Autodesk Inventor part; units mm, degrees
ref_plane "YZ Plane" through (0, 0, 0) normal (1, 0, 0) x (0, 1, 0)
ref_plane "XZ Plane" through (0, 0, 0) normal (0, 1, 0) x (-1, 0, 0)
ref_plane "XY Plane" through (0, 0, 0) normal (0, 0, 1) x (1, 0, 0)
sketch "Sketch1" plane through (0, 0, 0) normal (0, 1, 0) x (-1, 0, 0)
  line L0 (0, 225) -> (0, -225) construction
  line L1 (5, 225) -> (5, -225)
  line L2 (-5, -225) -> (-5, 225)
  arc A0 (5, 225) -> (-5, 225) centre (0, 225) ccw
  arc A1 (-5, -225) -> (5, -225) centre (0, -225) ccw
  circle A2 centre (0, 0) radius 2.5
  dimension "d0" = 450
  dimension "d1" = 10
  dimension "d2" = 5
extrude "Extrusion1" add sketch "Sketch1" along normal blind 10 contours L1 A1 L2 A0 | A2
sketch "Sketch2" plane through (0, 0, 0) normal (0, -1, 0) x (1, 0, 0)
  circle A0 centre (0, 0) radius 2.5
  dimension "d5" = 5
extrude "Extrusion2" add sketch "Sketch2" along normal blind 5
sketch "Sketch3" plane through (0, 10, 0) normal (0, 1, 0) x (1, 0, 0)
  line L0 (-5, 225) -> (-5, -225)
  arc A0 (-5, -225) -> (5, -225) centre (0, -225) ccw
  line L1 (5, -225) -> (5, 225)
  arc A1 (5, 225) -> (-5, 225) centre (0, 225) ccw
  circle A2 centre (0, -225) radius 5
  circle A3 centre (0, 225) radius 5
  line L2 (-5, -230) -> (5, -230)
  line L3 (5, -230) -> (5, -220)
  line L4 (5, -220) -> (-5, -220)
  line L5 (-5, -220) -> (-5, -230)
  line L6 (-5, 225) -> (-5, -225)
  line L7 (-5, 220) -> (5, 220)
  line L8 (5, 220) -> (5, 230)
  line L9 (5, 230) -> (-5, 230)
  line L10 (-5, 230) -> (-5, 220)
  point P0 (0, 0)
  point P1 (5, 225)
  point P2 (5, -225)
  point P3 (-5, -225)
  point P4 (0, 230)
  point P5 (5, 225)
  point P6 (-5, -225)
  point P7 (0, -230)
  point P8 (5, -225)
  dimension "d8" = 10
  dimension "d9" = 10
extrude "Extrusion3" add sketch "Sketch3" against normal blind 20 contours L10 L9 A1 | A1 A3 | L9 L8 A1 | A2 A0 | A0 L2 L5 | A0 L3 L2
properties part number "McCrea_otočka_walle"
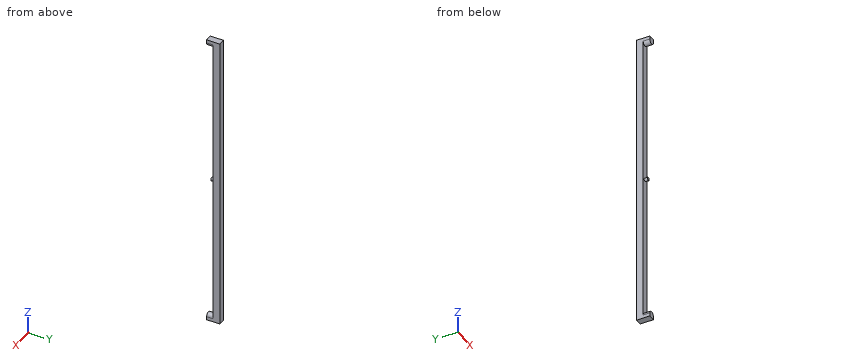
CAD build for the part. Positions are in the model's coordinates, mm. Round coordinates to 2 decimals unless told otherwise and drop trailing zeros. Order: outer loops, then holes, each group sorted by start corner. A loop starts at its lowest first (then second) coordinate and runs counter-clockwise, first axis right, second up.
Item 1: Probe line 1 along Y through (x, z) = (3, -87.5); line 2 along Z through (x, y) = (-2.25, -0.75); line 3 along Z through (x, y) = (4, -8.5). List the from-to ranges inside material, lowest first.
Item 2: Saw through at A-A on x = 0. Write the cut outline in (y, z).
Item 3: Saw through at B-B on z = 52. Write the cut outline in (x, y).
Item 4: Pin check, flat tips, straight feed: pin 1 (5 mm diameter, centred on x = -0.5, z = 27, fed in from -Y); pin 2 (2.5 mm diameter, centred on x = -1, z = 1, fed in from -Y). Stop position of each tip, or through.
Reported:
1. line 1: y = 0 to 10
1. line 2: z = -230 to -220.53, -1.09 to 1.09, 220.53 to 230
1. line 3: z = -230 to -222, 222 to 230
2. outline: (-10, -230) - (10, -230) - (10, 230) - (-10, 230) - (-10, 220) - (0, 220) - (0, 2.5) - (-5, 2.5) - (-5, -2.5) - (0, -2.5) - (0, -220) - (-10, -220) - close
3. outline: (-5, 0) - (5, 0) - (5, 10) - (-5, 10) - close
4. pin 1: stops at y = 0
4. pin 2: stops at y = -5
